Autodesk Inventor part; units mm, degrees
ref_plane "YZ Plane" through (0, 0, 0) normal (1, 0, 0) x (0, 1, 0)
ref_plane "XZ Plane" through (0, 0, 0) normal (0, 1, 0) x (-1, 0, 0)
ref_plane "XY Plane" through (0, 0, 0) normal (0, 0, 1) x (1, 0, 0)
sketch "Sketch1" plane through (0, 0, 0) normal (0, 1, 0) x (-1, 0, 0)
  line L0 (0, 0) -> (21.0058, 0)
  line L1 (21.0058, 0) -> (21.0058, -51.308)
  line L2 (21.0058, -51.308) -> (0, -51.308)
  line L3 (0, -51.308) -> (0, 0)
  line L4 (21.0058, -51.308) -> (19.8628, -51.308)
  line L5 (19.8628, -51.308) -> (19.8628, -50.292)
  line L6 (19.8628, -50.292) -> (21.0058, -50.292)
  line L7 (21.0058, -50.292) -> (21.0058, -51.308)
  line L8 (21.0058, -25.654) -> (0, -25.654)
  line L9 (10.5029, -51.308) -> (10.5029, 0)
  line L10 (19.8628, 0) -> (19.8628, -1.016)
  line L11 (19.8628, -1.016) -> (21.0058, -1.016)
  line L12 (1.143, -51.308) -> (1.143, -50.292)
  line L13 (1.143, -50.292) -> (0, -50.292)
  line L14 (1.143, -1.016) -> (0, -1.016)
  line L15 (1.143, 0) -> (1.143, -1.016)
  line L16 (19.8628, -1.016) -> (19.8628, -50.292)
  line L17 (19.8628, -50.292) -> (18.7198, -50.292)
  line L18 (18.7198, -50.292) -> (18.7198, -1.016)
  line L19 (18.7198, -1.016) -> (19.8628, -1.016)
  line L20 (1.143, -1.016) -> (1.143, -50.292)
  line L21 (1.143, -50.292) -> (2.286, -50.292)
  line L22 (2.286, -50.292) -> (2.286, -1.016)
  line L23 (2.286, -1.016) -> (1.143, -1.016)
  line L24 (21.0058, 0) -> (17.1958, 0)
  line L25 (17.1958, 0) -> (17.1958, -0.9398)
  line L26 (17.1958, -0.9398) -> (21.0058, -0.9398)
  line L27 (21.0058, -0.9398) -> (21.0058, 0)
  line L28 (17.1958, -0.9398) -> (15.2908, -0.9398)
  line L29 (15.2908, -0.9398) -> (15.2908, -2.8448)
  line L30 (15.2908, -2.8448) -> (17.1958, -2.8448)
  line L31 (17.1958, -2.8448) -> (17.1958, -0.9398)
  circle A0 centre (16.2433, -1.8923) radius 0.9525
  circle A1 centre (4.7625, -1.8923) radius 0.9525
  line L32 (21.0058, -51.308) -> (0, -51.308)
  line L33 (0, -51.308) -> (0, -50.165)
  line L34 (0, -50.165) -> (21.0058, -50.165)
  line L35 (21.0058, -50.165) -> (21.0058, -51.308)
  line L36 (21.0058, -50.165) -> (17.1958, -50.165)
  line L37 (17.1958, -50.165) -> (15.2908, -50.165)
  line L38 (15.2908, -50.165) -> (15.2908, -48.26)
  line L39 (15.2908, -48.26) -> (17.1958, -48.26)
  line L40 (17.1958, -48.26) -> (17.1958, -50.165)
  circle A2 centre (16.2433, -49.2125) radius 0.9525
  circle A3 centre (4.7625, -49.2125) radius 0.9525
  point P0 (19.8628, -50.165)
  point P1 (18.7198, -50.165)
  point P2 (2.286, -50.165)
  point P3 (1.143, -50.165)
  dimension "d0" = 21.0058
  dimension "d1" = 51.308
  dimension "d2" = 1.143
  dimension "d3" = 1.016
  dimension "d4" = 1.143
  dimension "d7" = 3.81
  dimension "d8" = 0.9398
  dimension "d9" = 1.905
  dimension "d10" = 1.905
  dimension "d11" = 1.143
  dimension "d12" = 3.81
  dimension "d13" = 1.905
  dimension "d14" = 1.905
extrude "Extrusion1" add sketch "Sketch1" along normal blind 1.016 contours L0 L15 L14 L3 | L0 L9 L8 L22 L23 L15 | L14 L20 L8 L3 | L31 A0 L28 | L0 L25 L26 L10 L19 L18 L8 L9 | L8 L20 L34 L3 | L0 L10 L26 L25 | L9 L34 L22 L8 | L8 L18 L34 L40 L39 L38 L9 | L34 L20 L13 L3 | L0 L1 L26 L10 | L34 L18 L17 L5 L2 L9 | L9 L2 L12 L21 L22 L34 | L34 L22 L21 L20 | L13 L12 L2 L3 | L26 L1 L11 L10 | A0 L29 L28 | L31 L30 A0 | L16 L11 L1 L8 | L8 L1 L34 L16 | L34 L16 L17 L18 | L38 A2 L34 | A0 L30 L29 | L34 L1 L6 L16 | L34 A2 L40 | L5 L6 L1 L2 | L38 L39 A2 | A2 L39 L40
sketch "Sketch2" plane through (0, 1.016, 0) normal (0, 1, 0) x (1, 0, 0)
  line L0 (0, 51.308) -> (-21.0058, 51.308)
  line L1 (-10.5029, 51.308) -> (-14.2875, 51.308)
  line L2 (-14.2875, 51.308) -> (-14.2875, 49.2125)
  line L3 (-14.2875, 49.2125) -> (-10.5029, 49.2125)
  line L4 (-10.5029, 49.2125) -> (-10.5029, 51.308)
  line L5 (-21.0058, 51.308) -> (0, 51.308)
  line L6 (-6.7183, 51.308) -> (-6.7183, 49.2125)
  line L7 (-6.7183, 49.2125) -> (-10.5029, 49.2125)
  point P0 (0, 0)
extrude "Extrusion2" add sketch "Sketch2" along normal blind 2.54
sketch "Sketch3" plane through (-14.2875, 1.016, -49.2125) normal (0, 0, 1) x (1, 0, 0)
  line L0 (0, 2.54) -> (7.5692, 2.54)
  line L1 (7.5692, 0) -> (0, 0)
  line L2 (0, 2.54) -> (7.5692, 2.54)
  line L3 (7.5692, 2.54) -> (7.5692, 0)
  line L4 (7.5692, 0) -> (0, 0)
  line L5 (0, 0) -> (0, 2.54)
  point P0 (14.2875, -1.016)
extrude "Extrusion3" add sketch "Sketch3" along normal blind 2.54
properties part number "RaspPi-Pico"
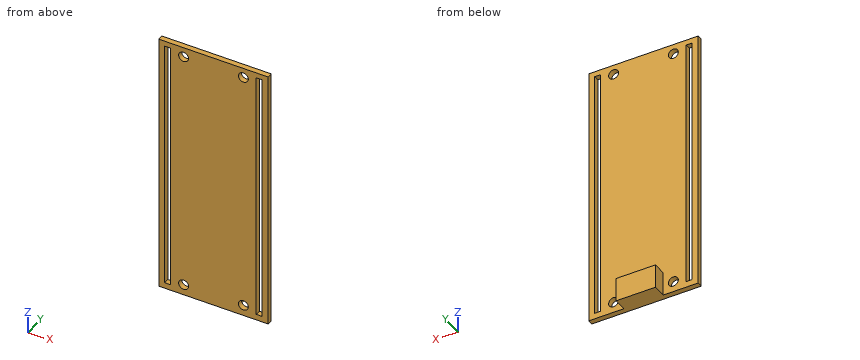
Check sheet for the modelled part. Datum: model origin and axes. Units: mm. Give positions to 0.01 mm unless a question says otherwise; leave off trailing zeros. Write each loop counter-clockwise with the first axis right and the second up, starting at its lowest first coordinate (ties: lowest second). Pieces come first, ordered by that corner, then holes. Notation, with made-up numbers: (-34, 76.25) -> (-17, 76.25) arc R12 ccw to (-17, 93.25) -> close; hole circle Ø9 at (2, 29.5). An arc over 180 degrees is marked (long way). Use CSV: the item, a comma, the result in double quotes. Start each with the question number.
Q1. Scan lines: line 1 along X through (y, z) = (0.3, -44.5); line 2 along Z through (x, y) = (-1.75, 0.8) (3 decimals); line 3 along Y through (x, z) = (-20, -20). Record each from-to range of solid material in increasing order.
Q2. Cross-section at A-A on z = -20.5. Enter the section's corners in (x, y), and give its area (3 significant figures).
Q3. Cross-section at D-D on x = -17.75. Enter the section's corners in (y, z).
Q4. Cross-section at C-C on y = 1.8. Enter the section's corners in (x, z), and give its area (3 significant figures).
Q5. Cross-section at B-B on x = -12. Enter the section's corners in (y, z), and give its area (3 significant figures).
Q6. Depth check by flat-ended pin: P1, Ø10, axis at x = -3, z = -33.5, coming from the +Y side; P2, Ø3, axis at x = -15, z = -42.5, coming from the -Y side; P3, Ø1.3, axis at x = -11, y = 2.5, coming from the +Z side. Enter the tip coordinate at first touch or a pass-through.
Working result:
1,line 1,"x = -21.01 to -19.86, -18.72 to -2.29, -1.14 to 0"
1,line 2,"z = -51.308 to -50.165, -1.016 to 0"
1,line 3,"y = 0 to 1.02"
2,outline,"(-21.01, 0) -> (-19.86, 0) -> (-19.86, 1.02) -> (-21.01, 1.02) -> close; (-18.72, 0) -> (-2.29, 0) -> (-2.29, 1.02) -> (-18.72, 1.02) -> close; (-1.14, 0) -> (0, 0) -> (0, 1.02) -> (-1.14, 1.02) -> close"
2,area,"19.0 mm^2"
3,outline,"(0, -51.31) -> (1.02, -51.31) -> (1.02, 0) -> (0, 0) -> close"
4,outline,"(-14.29, -51.31) -> (-6.72, -51.31) -> (-6.72, -46.67) -> (-14.29, -46.67) -> close"
4,area,"35.1 mm^2"
5,outline,"(0, -51.31) -> (3.56, -51.31) -> (3.56, -46.67) -> (1.02, -46.67) -> (1.02, 0) -> (0, 0) -> close"
5,area,"63.9 mm^2"
6,P1,"stops at y = 1.02"
6,P2,"stops at y = 0"
6,P3,"stops at z = -46.67"
